For this review, take the finished solid that the model builds, in its own axes (mm). A direction names the side the tool comes from. Give positions to 0.01 mm unless a question says otherwise; leave off trailing zeros. Loops run counter-clockwise (first coordinate to the right, second up) from the corner with the lowest first, then second, coordinate; pieces in that order, holes last.
```python
from build123d import *

# Parameters (mm, degrees)
F1_DEPTH = 12.7
F3_D     = 7.5946
F5_DEPTH = 25.4


with BuildPart() as f1:
    # F0 (on Front) → F1 (new body)
    with BuildSketch(Plane.XZ):
        Polygon((-13.766902, 0), (0, 0), (0, 8.422106), (-11.661377, 8.422106), (-20.245446, 3.401235), (-21.217227, -4.53498), align=None)
        Polygon((0, 8.422106), (0, 0), (7.774252, -2.105526), (20.731336, -17.654028), (23.386621, -10.155125), (11.661377, 4.858907), align=None)
    extrude(amount=F1_DEPTH)

    # F3 (through all)
    with Locations(Plane.XZ.offset(12.7)):
        with Locations((15.946049, -7.273637)):
            Hole(F3_D / 2)

    # F4 (on face) → F5 (cut)
    with BuildSketch(Plane.XZ.offset(12.7)):
        with BuildLine():
            ThreePointArc((21.587126, -7.850894), (19.681214, -11.027735), (16.154281, -12.161563))
            Line((16.154281, -12.161563), (20.731336, -17.654028))
            Line((20.731336, -17.654028), (23.386621, -10.155125))
            Line((23.386621, -10.155125), (21.587126, -7.850894))
        make_face()
    extrude(amount=-F5_DEPTH, mode=Mode.SUBTRACT)


solid = f1.part
```
Q1. Machinability: for faces 1 (the flat face through (15.66, -6.26, -11.57)), 2 (the flat face through (-17.544, -6.261, -2.299)), which of the approach directions +Z, -Z, +X, -X, +Y, -Y give a long, thin tool a straight path to every point of the face, cutting with its end or side? Answer none if there is none.
Answers:
face 1: -Z, -X, +Y, -Y
face 2: -Z, +Y, -Y
Q2. Consider section D-D on z = 6.5. Give the boundary of the cut face in (x, y).
Answers:
outline: (-14.95, -12.7) - (6.29, -12.7) - (6.29, 0) - (-14.95, 0) - close
Q3. For probe 1 along X at (y, z) = (-10, -3.25); probe 2 along Z at (x, y) = (-1.5, -7.5); probe 3 along X at (y, z) = (-8.5, -6.75), list the stretches that pass through material, from the lowest coordinate up.
Answers:
probe 1: x = -21.06 to -19.11, 8.73 to 17.99
probe 2: z = 0 to 8.42
probe 3: x = 11.64 to 12.19, 19.71 to 20.73
Q4. Consider section C-C on x = -2.5. Give the boundary of the cut face in (y, z), plus the area to 3 significant figures.
Answers:
outline: (-12.7, 0) - (0, 0) - (0, 8.42) - (-12.7, 8.42) - close
area: 107 mm2
Q5. Mouldability with a two-part tool opening along X and no side actions: class faces 3 (the flat face through (9.93, -6.26, -4.69)), 4 (the flat face through (-20.725, -6.261, -0.511)), 5 (the flat face through (-2, 0, 3)) as +X half, -X half, draft (parallel to the pull), parting line (faces both ways), or undercut.
Answers:
face 3: undercut
face 4: -X half
face 5: draft
Q6. Consider section B-B on x = 18. Give the boundary of the cut face in (y, z).
Answers:
outline: (-12.7, -11.92) - (0, -11.92) - (0, -10.47) - (-12.7, -10.47) - close; (-12.7, -4.08) - (0, -4.08) - (0, -3.26) - (-12.7, -3.26) - close
Q7. Consider section A-A on y = -9.75. Give the boundary of the cut face in (x, z).
Answers:
outline: (-21.22, -4.53) - (-13.77, 0) - (0, 0) - (7.77, -2.11) - (12.15, -7.36) arc R3.8 cw (long way) to (15.18, -10.99) - (16.15, -12.16) arc R5.26 ccw to (21.59, -7.85) - (11.66, 4.86) - (0, 8.42) - (-11.66, 8.42) - (-20.25, 3.4) - close
Q8. For pin 1 Ø4 at (x, y) = (-10, -7.5) entering from -Z, flat-tipped, find the tip position at first contact; note if it passes through.
Answers:
pin 1: stops at z = 0
